Could you check a few things on this drawing? It's one solid part, dimensions in mm from its lowest x, y, z. Round coordinates to 2 decimals unless told otherwise and drop trailing zeros. Write each loop counter-clockwise with the first axis right and the second up, starting at its lowest first coordinate (ties: lowest second). Pieces come first, ordered by that corner, then holes. Notation, with made-up numbers: (-25, 19.25) -> (11, 19.25) arc R27 ccw to (11, 38.25) -> close; hole circle Ø11 at (-10, -19). An arc over 180 degrees is marked (long way). Answer in a Markdown table with one row per item. Add a question column.
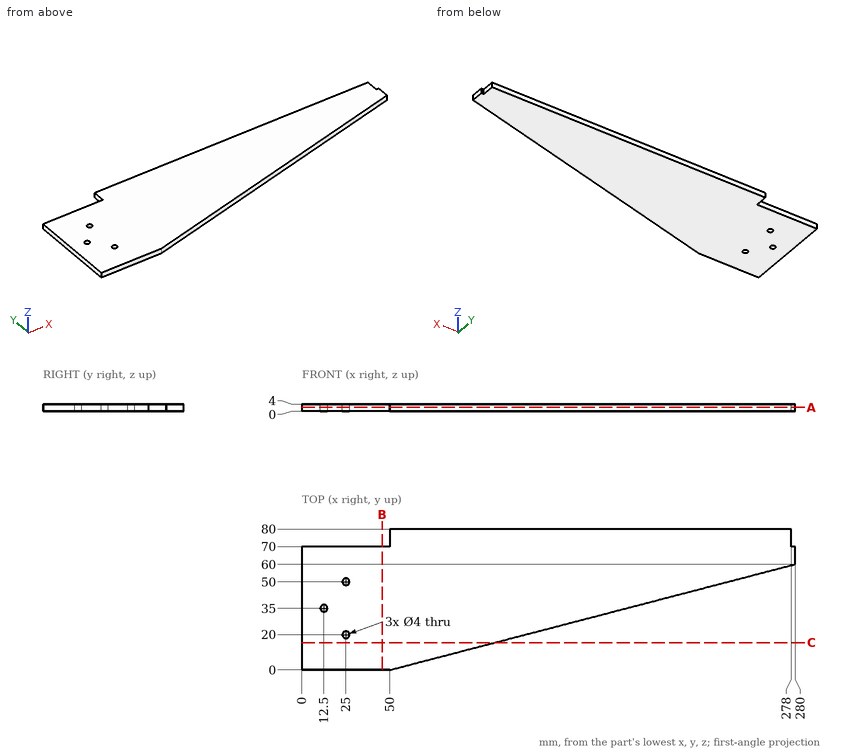
(1) Suppose I cut it at C-C, the plane y = 15.5. Please give me the cut outline in (x, z), then the cut area to 3 significant figures.
(2) Suppose I cut it at B-B, the plane x = 45.5. Please give me the cut outline in (y, z).
(3) For P1, Ø1.5, axis at x = 170.5, z = 1, coming from the -Y side; P2, Ø1.5, axis at x = 221, z = 3.5, coming from the -Y side; P3, Ø0.6, axis at x = 279.5, z = 2.5, coming from the +Y side, each with a flat end and sliding along its axis, tell me the tip position at first contact or that it passes through.
(4) Suppose I cut it at A-A, the plane z = 2.1. Please give me the cut outline in (x, y), then the cut area to 3 significant figures.
(5) I need wall thicknesses on L1, parallel to Y at x = 25, z = 2.7; L2, parallel to Y at x = 12.5, z = 1.5; L3, parallel to X at y = 73.5, z = 2.5. Which ranges of each line are inside material? Lowest first, please.
Response:
| question | item | result |
|---|---|---|
| 1 | outline | (0, 0) -> (109.42, 0) -> (109.42, 4) -> (0, 4) -> close |
| 1 | area | 438 mm² |
| 2 | outline | (0, 0) -> (70, 0) -> (70, 4) -> (0, 4) -> close |
| 3 | P1 | y = 31.24 |
| 3 | P2 | y = 44.41 |
| 3 | P3 | y = 70 |
| 4 | outline | (0, 0) -> (50, 0) -> (280, 60) -> (280, 70) -> (278, 70) -> (278, 80) -> (50, 80) -> (50, 70) -> (0, 70) -> close; hole circle Ø4 at (12.5, 35); hole circle Ø4 at (25, 20); hole circle Ø4 at (25, 50) |
| 4 | area | 14,900 mm² |
| 5 | L1 | 0 to 18, 22 to 48, 52 to 70 |
| 5 | L2 | 0 to 33, 37 to 70 |
| 5 | L3 | 50 to 278 |
